For this review, use the dimensioned drawing (mm, ordinates from the lowest corner) and the shaded views. A direction names the side the tool comes from. Give positions to 0.01 mm unless a question says otherwise; leave off trailing zeros. Loops run counter-clockwise (first coordinate to the right, second up) from the corner with the lowest first, then second, coordinate; pieces in that order, holes last. Notation, with made-up numbers: M 75.25,73.25 L 114.25,73.25 A21 cw 114.25,92.25 Z; hole C 33.5,4 d1. An arc over 180 degrees is marked long. Use a Markdown table: item, result. Add a question column.
(1) Add section A-A, the plane y = 20. Give the boundary of the cut face in (x, z), then the cut area to 3 significant figures.
(2) Add section D-D, the plane x = 157.5. Give the boundary of the cut face in (y, z).
(3) Insertion check: pin 1 Ø6 at (x, z) = (154, 25) entering from -Y; pin 2 Ø12 at (y, z) = (19.5, 17.5) entering from -X; pin 3 Ø2 at (x, y) = (59, 18.5) entering from -Z; pin 4 Ø6 at (x, z) = (79.5, 16) entering from -Y (3 decimals). Each pin has a flat end and moves straight along its axis. Give the tip position at first contact, or say it passes through.
(4) For probe 1 along Z at (x, y) = (111, 16); probe 2 along X at (y, z) = (24, 37); probe 3 along X at (y, z) = (22, 38), list the stretches that pass through material, from the lowest coordinate up.
(5) For the marked faces 1, 2 and 3, list the 3-axis set-ups (+Z, -Z, +X, -X, +Y, -Y) from which the entire face can be reached by the end or side of a thin tool; tool diameter is ignored.
(6) Add section C-C, the plane x = 120. Give the boundary of the cut face in (y, z), then the cut area to 3 significant figures.
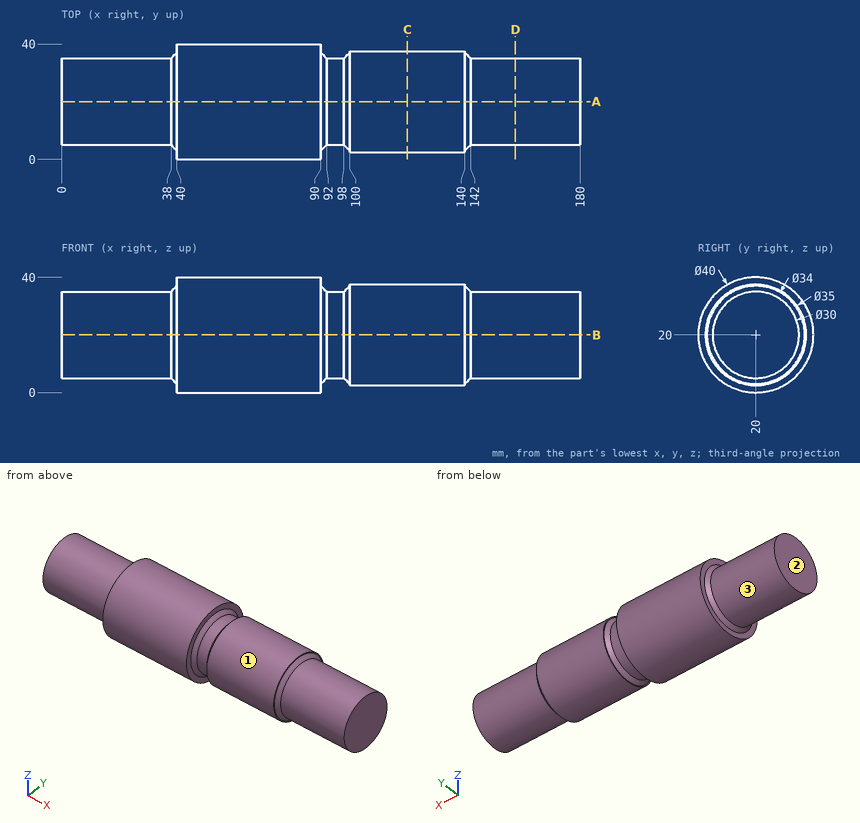
Established:
| question | item | result |
|---|---|---|
| 1 | outline | M 0,5 L 38,5 L 40,3 L 40,0 L 90,0 L 90,3 L 92,5 L 98,5 L 100,3 L 100,2.5 L 140,2.5 L 140,3 L 142,5 L 180,5 L 180,35 L 142,35 L 140,37 L 140,37.5 L 100,37.5 L 100,37 L 98,35 L 92,35 L 90,37 L 90,40 L 40,40 L 40,37 L 38,35 L 0,35 Z |
| 1 | area | 6,120 mm^2 |
| 2 | outline | C 20,20 d30 |
| 3 | pin 1 | y = 5.13 |
| 3 | pin 2 | x = 0 |
| 3 | pin 3 | z = 0.01 |
| 3 | pin 4 | y = 0.025 |
| 4 | probe 1 | 2.96 to 37.04 |
| 4 | probe 2 | 40 to 90, 100 to 140 |
| 4 | probe 3 | 40 to 90 |
| 5 | face 1 | +X |
| 5 | face 2 | +Z, -Z, -X, +Y, -Y |
| 5 | face 3 | -X |
| 6 | outline | C 20,20 d35 |
| 6 | area | 962 mm^2 |
